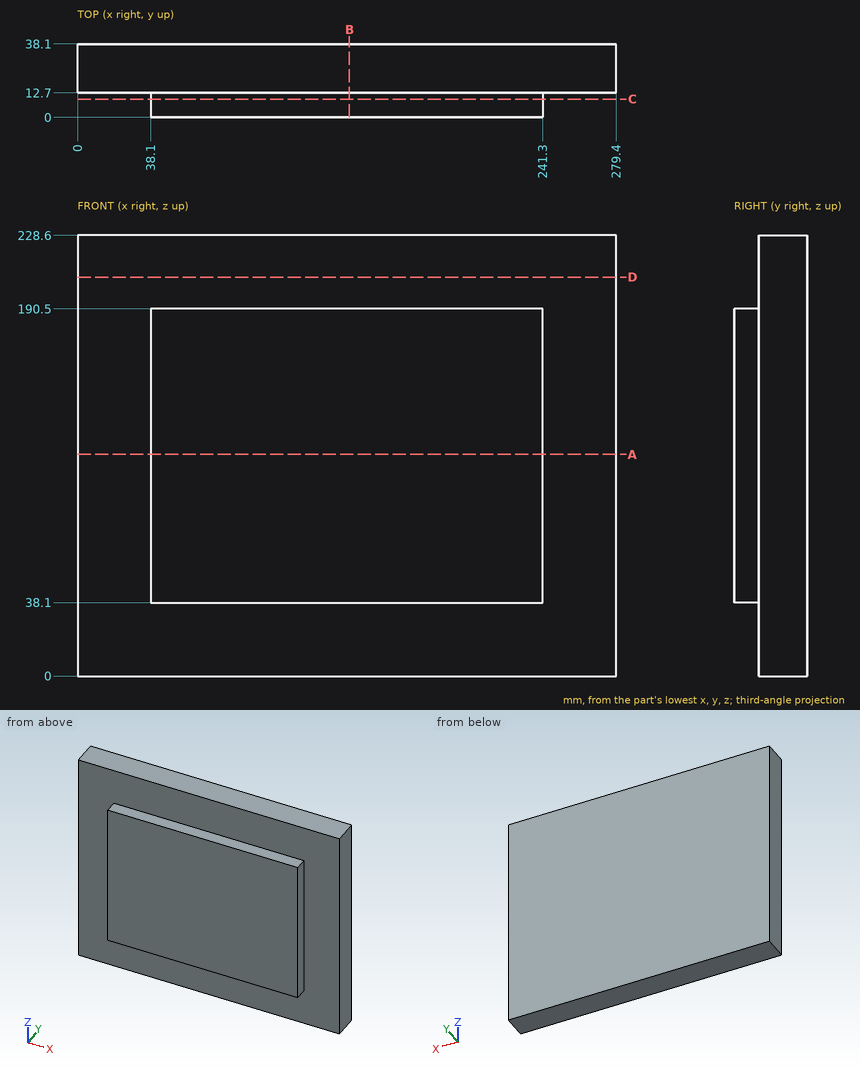
Input: dimensioned drawing with shaded views. Units: mm. Origin: part minimum x, y, z. Coordinates: 2 decimals unless noted, no trailing zeros. Loops run counter-clockwise (first coordinate to the right, second up) from the corner with the lowest first, then second, coordinate; pieces in that order, holes last. Notation, with made-up numbers: (66.25, -3.5) -> (125.25, -3.5) arc R19 cw to (125.25, 3.5) -> close; hole circle Ø11 at (-10, -15). An arc over 180 degrees is marked (long way). Use a Markdown table: item, result. Add a question column.
(1) Section query C-C, the plane y = 9.5. Return loops of the section in (x, z).
(2) Section query A-A, the plane z = 115. Return loops of the section in (x, y), plus the area to 3 significant figures.
(3) Section query D-D, the plane z = 207. Return loops of the section in (x, y), plus the area to 3 significant figures.
(4) Line query: line 1 along Z through (x, y) = (86.5, 12); line 2 along Y through (x, z) = (98.5, 29); line 3 along X through (y, z) = (7, 185). Output: solid intervals per line, ascending.
(5) Section query B-B, the plane x = 141. Return loops of the section in (y, z), plus the area to 3 significant figures.
(6) Pin query (flat end, axial travel): pin 1 Ø8 at (y, z) = (26.5, 93.5) entering from -X; pin 2 Ø6.5 at (x, y) = (105.5, 4.5) entering from +Z. Return the tip coordinate at first contact, or that it passes through.
Answer:
| question | item | result |
|---|---|---|
| 1 | outline | (38.1, 38.1) -> (241.3, 38.1) -> (241.3, 190.5) -> (38.1, 190.5) -> close |
| 2 | outline | (0, 12.7) -> (38.1, 12.7) -> (38.1, 0) -> (241.3, 0) -> (241.3, 12.7) -> (279.4, 12.7) -> (279.4, 38.1) -> (0, 38.1) -> close |
| 2 | area | 9,680 mm^2 |
| 3 | outline | (0, 12.7) -> (279.4, 12.7) -> (279.4, 38.1) -> (0, 38.1) -> close |
| 3 | area | 7,100 mm^2 |
| 4 | line 1 | z = 38.1 to 190.5 |
| 4 | line 2 | y = 12.7 to 38.1 |
| 4 | line 3 | x = 38.1 to 241.3 |
| 5 | outline | (0, 38.1) -> (12.7, 38.1) -> (12.7, 0) -> (38.1, 0) -> (38.1, 228.6) -> (12.7, 228.6) -> (12.7, 190.5) -> (0, 190.5) -> close |
| 5 | area | 7,740 mm^2 |
| 6 | pin 1 | stops at x = 0 |
| 6 | pin 2 | stops at z = 190.5 |
